```python
from build123d import *

# Parameters (mm, degrees)
SKETCH_W        = 47.5
SKETCH_H        = 39
PAD_DEPTH       = 34
SKETCH001_R     = 13.5
SKETCH001_R_2   = 2
POCKET_DEPTH    = 40
SKETCH002_R     = 2
POCKET001_DEPTH = 20


with BuildPart() as part:
    # Sketch → Pad (new body)
    with BuildSketch(Plane.XY):
        with Locations((0, 19.5)):
            Rectangle(SKETCH_W, SKETCH_H)
    extrude(amount=PAD_DEPTH)

    # Sketch001 → Pocket (cut)
    with BuildSketch(Plane.XY.offset(34)):
        with Locations((0, 19.5)):
            Circle(SKETCH001_R)
        with Locations((-18.5, 19.5)):
            Circle(SKETCH001_R_2)
        with Locations((18.5, 19.5)):
            Circle(SKETCH001_R_2)
        with Locations((13.081476, 6.418525)):
            Circle(SKETCH001_R_2)
        with Locations((13.081476, 32.581475)):
            Circle(SKETCH001_R_2)
        with Locations((-13.081476, 6.418525)):
            Circle(SKETCH001_R_2)
        with Locations((-13.081476, 32.581475)):
            Circle(SKETCH001_R_2)
    extrude(amount=-POCKET_DEPTH, mode=Mode.SUBTRACT)

    # Sketch002 → Pocket001 (cut)
    with BuildSketch(Plane.XZ):
        with Locations((18.75, 4.5)):
            Circle(SKETCH002_R)
        with Locations((-18.75, 4.5)):
            Circle(SKETCH002_R)
        with Locations((18.75, 26)):
            Circle(SKETCH002_R)
        with Locations((-18.75, 26)):
            Circle(SKETCH002_R)
    extrude(amount=-POCKET001_DEPTH, mode=Mode.SUBTRACT)


solid = part.part
```
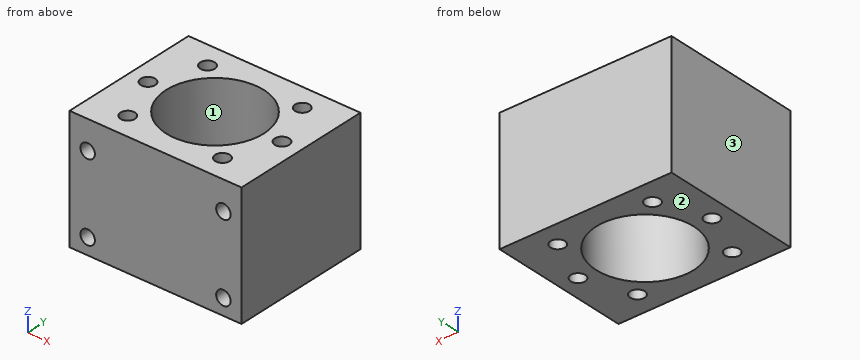
Verification items for the finished model (mm, model axes). Face numbers are marked on the shaded views. Round coordinates to 2 decimals unless told otherwise and drop trailing zeros. Write each loop counter-clockwise with the first axis right and the second up, starting at its lowest first coordinate (ties: lowest second). Pieces come first, ordered by that corner, then holes.
1. Section check C-C on y = 2.5. Enter the section's corners in (x, z), plus the area to 3 significant figures.
2. Section check A-A on x = 0. Enter the section's corners in (y, z).
3. Section check B-B on y = 9. Enter the section's corners in (x, z), plus the area to 3 significant figures.
4. Section check D-D on x = 18.75. Enter the section's corners in (y, z).
5. Gauge pin test, flat end, axial feed: P1, Ø2.5, axis at x = 13.08, y = 6.42, coming from the +Z side. Record the tip position at first contact, or that the pin passes through.
6. Scan lines: L1, parallel to Z at x = -18.75, y = 11.5; L2, parallel to X at y = 31.5, z = 26; L3, parallel to Y at x = 0, z = 18. Record each from-to range of solid material in increasing order.
7. Draft check along X on the marked faces 1, 2 and 3. Enter one of: +X half, -X half, draft (parallel to the pull), parting line (faces both ways), or undercut.
Answer:
1. outline: (-23.75, 0) - (23.75, 0) - (23.75, 34) - (-23.75, 34) - close; hole circle Ø4 at (-18.75, 4.5); hole circle Ø4 at (-18.75, 26); hole circle Ø4 at (18.75, 4.5); hole circle Ø4 at (18.75, 26)
1. area: 1,560 mm2
2. outline: (0, 0) - (6, 0) - (6, 34) - (0, 34) - close; (33, 0) - (39, 0) - (39, 34) - (33, 34) - close
3. outline: (-23.75, 0) - (-8.49, 0) - (-8.49, 34) - (-23.75, 34) - close; (8.49, 0) - (23.75, 0) - (23.75, 34) - (8.49, 34) - close; hole circle Ø4 at (-18.75, 4.5); hole circle Ø4 at (-18.75, 26); hole circle Ø4 at (18.75, 4.5); hole circle Ø4 at (18.75, 26)
3. area: 988 mm2
4. outline: (0, 0) - (17.52, 0) - (17.52, 2.5) - (0, 2.5) - close; (0, 6.5) - (17.52, 6.5) - (17.52, 24) - (0, 24) - close; (0, 28) - (17.52, 28) - (17.52, 34) - (0, 34) - close; (21.48, 0) - (39, 0) - (39, 34) - (21.48, 34) - close
5. P1: passes through
6. L1: z = 0 to 2.5, 6.5 to 24, 28 to 34
6. L2: x = -23.75 to -14.76, -11.4 to -6.18, 6.18 to 11.4, 14.76 to 23.75
6. L3: y = 0 to 6, 33 to 39
7. face 1: undercut
7. face 2: draft
7. face 3: -X half
